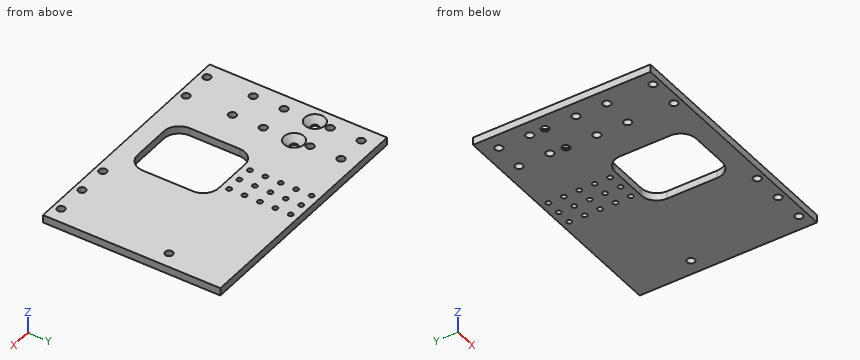
from build123d import *

# Parameters (mm, degrees)
SKETCH1_W               = 203.2
SKETCH1_H               = 146.05
BOSS_EXTRUDE1_DEPTH     = 6.35
CUT_EXTRUDE1_DEPTH      = 251.322122474
CUT_EXTRUDE1_DEPTH_BACK = 251.322122474
SKETCH2_R               = 3.175
CUT_EXTRUDE2_DEPTH      = 251.322122474
CUT_EXTRUDE2_DEPTH_BACK = 251.322122474
SKETCH3_R               = 2.032
CUT_EXTRUDE3_DEPTH      = 251.322122474
CUT_EXTRUDE3_DEPTH_BACK = 251.322122474
SKETCH4_W               = 57.15
SKETCH4_H               = 66.675
FILLET1_R               = 12.7
CHAMFER1_SIZE           = 5.08


with BuildPart() as part:
    # Sketch1 → Boss-Extrude1 (new body)
    with BuildSketch(Plane.XY):
        with Locations((101.6, 73.025)):
            Rectangle(SKETCH1_W, SKETCH1_H)
    extrude(amount=BOSS_EXTRUDE1_DEPTH)

    # Sketch2 → Cut-Extrude1 (cut, two sides: drawn at the far end of the back side and taken through both)
    with BuildSketch(Plane.XY.offset(6.35).offset(-CUT_EXTRUDE1_DEPTH_BACK)):
        with Locations((12.7, 133.35)):
            Circle(SKETCH2_R)
        with Locations((37.270330063, 133.35)):
            Circle(SKETCH2_R)
        with Locations((12.7, 107.904145464)):
            Circle(SKETCH2_R)
        with Locations((37.270330063, 107.904145464)):
            Circle(SKETCH2_R)
        with Locations((12.7, 95.25)):
            Circle(SKETCH2_R)
        with Locations((38.1, 95.25)):
            Circle(SKETCH2_R)
        with Locations((12.7, 69.85)):
            Circle(SKETCH2_R)
        with Locations((38.1, 69.85)):
            Circle(SKETCH2_R)
        with Locations((12.7, 44.45)):
            Circle(SKETCH2_R)
        with Locations((38.1, 44.45)):
            Circle(SKETCH2_R)
        with Locations((12.7, 6.35)):
            Circle(SKETCH2_R)
        with Locations((38.1, 6.35)):
            Circle(SKETCH2_R)
        with Locations((139.7, 6.35)):
            Circle(SKETCH2_R)
        with Locations((165.1, 6.35)):
            Circle(SKETCH2_R)
        with Locations((190.5, 6.35)):
            Circle(SKETCH2_R)
        with Locations((190.5, 95.25)):
            Circle(SKETCH2_R)
    extrude(amount=CUT_EXTRUDE1_DEPTH + CUT_EXTRUDE1_DEPTH_BACK, mode=Mode.SUBTRACT)

    # Sketch3 → Cut-Extrude2 (cut, two sides: drawn at the far end of the back side and taken through both)
    with BuildSketch(Plane.XY.offset(6.35).offset(-CUT_EXTRUDE2_DEPTH_BACK)):
        with Locations((95.25, 139.7)):
            Circle(SKETCH3_R)
        with Locations((107.95, 139.7)):
            Circle(SKETCH3_R)
        with Locations((82.55, 139.7)):
            Circle(SKETCH3_R)
        with Locations((107.95, 127)):
            Circle(SKETCH3_R)
        with Locations((95.25, 127)):
            Circle(SKETCH3_R)
        with Locations((82.55, 127)):
            Circle(SKETCH3_R)
        with Locations((107.95, 114.3)):
            Circle(SKETCH3_R)
        with Locations((95.25, 114.3)):
            Circle(SKETCH3_R)
        with Locations((82.55, 114.3)):
            Circle(SKETCH3_R)
        with Locations((107.95, 101.6)):
            Circle(SKETCH3_R)
        with Locations((95.25, 101.6)):
            Circle(SKETCH3_R)
        with Locations((82.55, 101.6)):
            Circle(SKETCH3_R)
        with Locations((107.95, 88.9)):
            Circle(SKETCH3_R)
        with Locations((95.25, 88.9)):
            Circle(SKETCH3_R)
        with Locations((82.55, 88.9)):
            Circle(SKETCH3_R)
    extrude(amount=CUT_EXTRUDE2_DEPTH + CUT_EXTRUDE2_DEPTH_BACK, mode=Mode.SUBTRACT)

    # Sketch4 → Cut-Extrude3 (cut, two sides: drawn at the far end of the back side and taken through both)
    with BuildSketch(Plane.XY.offset(6.35).offset(-CUT_EXTRUDE3_DEPTH_BACK)):
        with Locations((95.25, 49.2125)):
            Rectangle(SKETCH4_W, SKETCH4_H)
    extrude(amount=CUT_EXTRUDE3_DEPTH + CUT_EXTRUDE3_DEPTH_BACK, mode=Mode.SUBTRACT)

    # Fillet1
    fillet1_edges = [part.edges().sort_by_distance(p)[0] for p in [
        (66.675, 15.875, 3.175),
        (66.675, 82.55, 3.175),
        (123.825, 82.55, 3.175),
        (123.825, 15.875, 3.175),
    ]]
    fillet(fillet1_edges, radius=FILLET1_R)

    # Chamfer1
    chamfer1_edges = [part.edges().sort_by_distance(p)[0] for p in [
        (34.925, 95.25, 6.35),
        (9.525, 95.25, 6.35),
    ]]
    chamfer(chamfer1_edges, length=CHAMFER1_SIZE)


solid = part.part
Source: CAD feature listing. Evaluate the final solid. Frame: model axes, mm. Coordinates: 2 decimals unless noted, no trailing zeros. Order: outer loops, then holes, each group sorted by start corner. A loop starts at its lowest first (then second) coordinate and runs counter-clockwise, first axis right, second up. Notation, with made-up numbers: M 10.25,28 L 50.25,28 A24 cw 50.25,54 Z; hole C 35.5,16.25 d2. An arc over 180 degrees is marked long. Write each question's results on one line, items separated by ' | '. Start each with the question number.
Item 1: Cut plane C-C (y = 79). Return loops of the section in (x, z).
Item 2: Line query: probe 1 along X at (y, z) = (88.9, 1.5); probe 2 along X at (y, z) = (44.5, 5.25) (3 decimals); probe 3 along X at (y, z) = (133.35, 2) (3 decimals). Output: solid intervals per line, ascending.
Item 3: First-contact query: pin 1 Ø5.5 at (x, y) = (12.7, 6.35) entering from +Z (3 decimals); pin 2 Ø7.5 at (x, y) = (38.1, 95.25) entering from +Z (3 decimals). Flat tips, straight axial feed; report the tip coordinate or a pass-through.
Item 4: Cut plane B-B (y = 44.45). Return loops of the section in (x, z) (3 decimals).
Item 5: Cut plane A-A (x = 88.5). Return loops of the section in (y, z) (3 decimals).
Item 6: Cut plane D-D (z = 3.25). Count the separate pieces of the cut face and the enclosed holes in it, and give its area (3 significant figures).
Checked values:
1) outline: M 0,0 L 70.57,0 L 70.57,6.35 L 0,6.35 Z; M 119.93,0 L 203.2,0 L 203.2,6.35 L 119.93,6.35 Z
2) probe 1: x = 0 to 80.52, 84.58 to 93.22, 97.28 to 105.92, 109.98 to 203.2 | probe 2: x = 0 to 9.525, 15.875 to 34.925, 41.275 to 66.675, 123.825 to 203.2 | probe 3: x = 0 to 9.525, 15.875 to 34.095, 40.445 to 203.2
3) pin 1: passes through | pin 2: stops at z = 1.845
4) outline: M 0,0 L 9.525,0 L 9.525,6.35 L 0,6.35 Z; M 15.875,0 L 34.925,0 L 34.925,6.35 L 15.875,6.35 Z; M 41.275,0 L 66.675,0 L 66.675,6.35 L 41.275,6.35 Z; M 123.825,0 L 203.2,0 L 203.2,6.35 L 123.825,6.35 Z
5) outline: M 0,0 L 15.875,0 L 15.875,6.35 L 0,6.35 Z; M 82.55,0 L 146.05,0 L 146.05,6.35 L 82.55,6.35 Z
6) separate pieces: 1 | enclosed holes: 32 | area: 25,200 mm2
